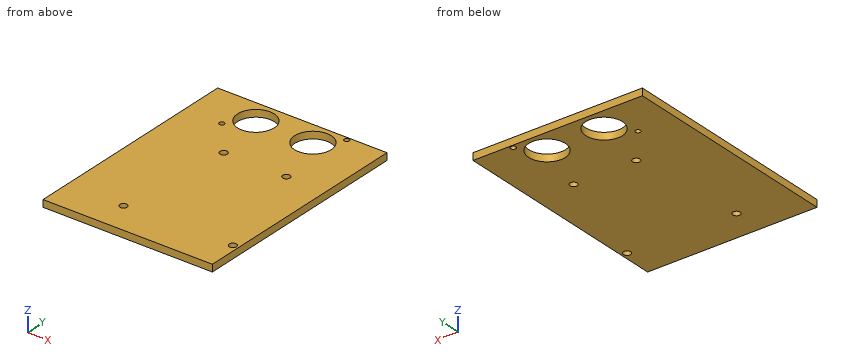
```python
from build123d import *

# Parameters (mm, degrees)
SKETCH2_W           = 76.2
SKETCH2_H           = 101.6
BOSS_EXTRUDE1_DEPTH = 3.175
SKETCH3_R           = 8.255
SKETCH3_R_2         = 1.143
CUT_EXTRUDE1_DEPTH  = 3.175
SKETCH6_R           = 1.651
CUT_EXTRUDE2_DEPTH  = 3.175


with BuildPart() as part:
    # Sketch2 → Boss-Extrude1 (new body)
    with BuildSketch(Plane.XY):
        with Locations((38.1, 50.8)):
            Rectangle(SKETCH2_W, SKETCH2_H)
    extrude(amount=BOSS_EXTRUDE1_DEPTH)

    # Sketch3 → Cut-Extrude1 (cut)
    with BuildSketch(Plane.XY.offset(3.175)):
        with Locations((25.273, 91.186)):
            Circle(SKETCH3_R)
        with Locations((50.927, 91.186)):
            Circle(SKETCH3_R)
        with Locations((59.269530294, 100.076)):
            Circle(SKETCH3_R_2)
        with Locations((16.851530294, 82.296)):
            Circle(SKETCH3_R_2)
    extrude(amount=-CUT_EXTRUDE1_DEPTH, mode=Mode.SUBTRACT)

    # Sketch6 → Cut-Extrude2 (cut)
    with BuildSketch(Plane(origin=(0, 0, 0), x_dir=(-1, 0, 0), z_dir=(0, 0, -1))):
        with Locations((-73.66, 15.24)):
            Circle(SKETCH6_R)
        with Locations((-25.4, 13.97)):
            Circle(SKETCH6_R)
        with Locations((-30.226, 66.04)):
            Circle(SKETCH6_R)
        with Locations((-58.42, 66.04)):
            Circle(SKETCH6_R)
    extrude(amount=-CUT_EXTRUDE2_DEPTH, mode=Mode.SUBTRACT)


solid = part.part
```
Here's how the part is built. I have some questions about the finished solid (model axes, mm). Coordinates: 2 decimals unless noted, no trailing zeros. Order: outer loops, then holes, each group sorted by start corner. A loop starts at its lowest first (then second) coordinate and runs counter-clockwise, first axis right, second up. Notation, with made-up numbers: M 87,58 L 146,58 A26 ccw 146,73 Z; hole C 20.25,44.25 d9. An arc over 180 degrees is marked long. Answer as a JSON object with one key per item and string values. Group by question number.
(1) For pin 1 (5 mm diameter, centred on x = 37, y = 62, fed in from -Z), with a flat end and sliding along its axis, tell me the tip position at first contact or that it passes through.
(2) I need wall thicknesses on probe 1 along Y at (x, z) = (73.66, 1.85); probe 2 along X at (y, z) = (86, 0.75); probe 3 along X at (y, z) = (95.5, 2). Which ranges of each line are inside material? Lowest first, please.
(3) Suppose I cut it at C-C, the plane x = 25.4. Please give me the cut outline in (y, z) (3 decimals).
(4) Suppose I cut it at D-D, the plane x = 48. Please give me the cut outline in (y, z) (3 decimals).
(5) Suppose I cut it at A-A, the plane y = 66.04. Please give me the cut outline in (x, z) (3 decimals), then the cut area to 3 significant figures.
(6) Suppose I cut it at B-B, the plane z = 1.7. State how many separate pieces and enclosed holes the cut face has, then the cut area to 3 significant figures.
Values found:
{
 "1": {"pin 1": "stops at z = 0"},
 "2": {"probe 1": "y = 0 to 13.59, 16.89 to 101.6", "probe 2": "x = 0 to 18.85, 31.7 to 44.5, 57.35 to 76.2", "probe 3": "x = 0 to 18.23, 32.31 to 43.89, 57.97 to 76.2"},
 "3": {"outline": "M 0,0 L 12.319,0 L 12.319,3.175 L 0,3.175 Z; M 15.621,0 L 82.932,0 L 82.932,3.175 L 15.621,3.175 Z; M 99.44,0 L 101.6,0 L 101.6,3.175 L 99.44,3.175 Z"},
 "4": {"outline": "M 0,0 L 83.467,0 L 83.467,3.175 L 0,3.175 Z; M 98.905,0 L 101.6,0 L 101.6,3.175 L 98.905,3.175 Z"},
 "5": {"outline": "M 0,0 L 28.575,0 L 28.575,3.175 L 0,3.175 Z; M 31.877,0 L 56.769,0 L 56.769,3.175 L 31.877,3.175 Z; M 60.071,0 L 76.2,0 L 76.2,3.175 L 60.071,3.175 Z", "area": "221 mm^2"},
 "6": {"separate pieces": "1", "enclosed holes": "8", "area": "7,270 mm^2"}
}
